Read the model definition and answer for the solid it produces. Units are mm, in the model's axes. A direction names the side the tool comes from. Coordinates: 2 decimals unless noted, no trailing zeros. Write each loop counter-clockwise with the first axis right and the second up, starting at its lowest first coordinate (ties: lowest second). Pieces come first, ordered by that corner, then holes.
(1) Which of the six approach directions +Z, -Z, +X, -X, +Y, -Y give full straight-line access (tool end or side, diameter ignored) to faces 1 (the flat face through (0, 49, 150)), 2 (the cylindrical face through (-44.292, 16.725, 76.05))?
(2) Given pin 1 (6.5 mm diameter, centred on y = 6.5, z = 76.5, fed in from +X); pin 2 (1.5 mm diameter, centred on y = 42.5, z = 96.5, fed in from -X); pin 3 (10 mm diameter, centred on x = 6.5, z = 133, fed in from -Y), each flat-ended and moving along its own axis, determine where each tip first touches the part or whether it passes through.
(3) Section C-C on x = 0 is taken. Write down the section's boundary in (y, z), then the cut area to 3 significant figures.
(4) The mould has two halves that part along X. Classify faces 3 (the cylindrical face through (44.304, 16.669, 76.05)), 4 (the cylindrical face through (-1.06, 49.49, 73.95)), 5 (the flat face through (-44.5, 8, 74)), 6 (the flat face through (0, 49, 0)): +X half, -X half, draft (parallel to the pull), parting line (faces both ways), or undercut.
(5) Section D-D on x = 18.5 is taken. Write down the section's boundary in (y, z).
(6) Find the intervals of material crossed by probe 1 along X at (y, z) = (2, 21); probe 2 along X at (y, z) = (30, 134.5); probe 3 along Y at (x, z) = (-1, 87), in increasing order.
(7) Section B-B on y = 6 is taken. Write down the section's boundary in (x, z).
Autodesk Inventor part; units mm, degrees
ref_plane "YZ Plane" through (0, 0, 0) normal (1, 0, 0) x (0, 1, 0)
ref_plane "XZ Plane" through (0, 0, 0) normal (0, 1, 0) x (-1, 0, 0)
ref_plane "XY Plane" through (0, 0, 0) normal (0, 0, 1) x (1, 0, 0)
sketch "Sketch1" plane through (0, 0, 0) normal (0, 0, 1) x (1, 0, 0)
  arc A0 (49.5, 0) -> (-49.5, 0) centre (0, 0) ccw
  arc A1 (47.5, 0) -> (-47.5, 0) centre (0, 0) ccw
  line L0 (47.5, 0) -> (49.5, 0)
  line L1 (-47.5, 0) -> (-49.5, 0)
  line L2 (-49.5, 0) -> (-44.5, 0)
  line L3 (-44.5, 0) -> (-44.5, 16.6132)
  line L4 (49.5, 0) -> (44.5, 0)
  line L5 (44.5, 0) -> (44.5, 16.6132)
  point P0 (-47.5, 0)
  dimension "d0" = 99
  dimension "d1" = 2
  dimension "d4" = 5
  dimension "d6" = 5
extrude "Extrusion1" add sketch "Sketch1" along normal blind 150
fillet "Fillet1" radius 2 4 edges at (-44.5, 0, 75) (-49.5, 0, 75) (44.5, 0, 75) (49.5, 0, 75)
fillet "Fillet2" radius 10 2 edges at (-44.5, 16.6132, 75) (44.5, 16.6132, 75)
equation "\"d1\" = 2 * extrusion_width"
equation "\"extrusion_width\" = 1"
properties part number "Parts-Tray-for-plasma-vessel"
Response:
1. face 1: +Z, +X, -X, +Y, -Y
1. face 2: +Z, -Z, -Y
2. pin 1: stops at x = 49.39
2. pin 2: stops at x = -26.59
2. pin 3: stops at y = 46.09
3. outline: (47.5, 0) - (49.5, 0) - (49.5, 150) - (47.5, 150) - close
3. area: 300 mm2
4. face 3: undercut
4. face 4: parting line
4. face 5: undercut
4. face 6: draft
5. outline: (43.75, 0) - (45.91, 0) - (45.91, 150) - (43.75, 150) - close
6. probe 1: x = -49.46 to -44.5, 44.5 to 49.46
6. probe 2: x = -39.37 to -36.83, 36.83 to 39.37
6. probe 3: y = 47.49 to 49.49
7. outline: (-49.14, 0) - (-44.5, 0) - (-44.5, 150) - (-49.14, 150) - close; (44.5, 0) - (49.14, 0) - (49.14, 150) - (44.5, 150) - close
